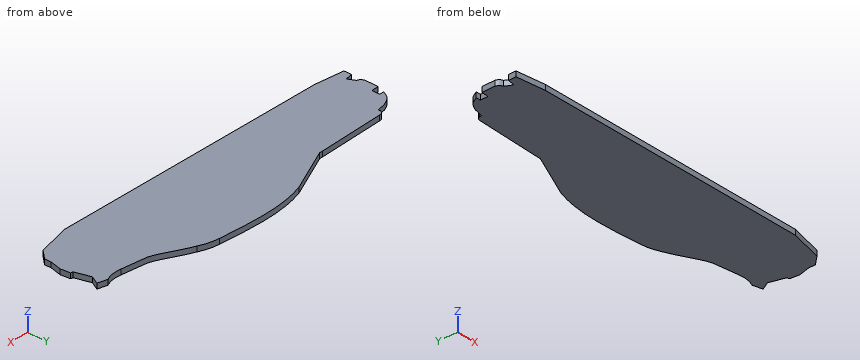
from build123d import *

# Parameters (mm, degrees)
BOSS_EXTRUDE1_DEPTH = 3.18


with BuildPart() as part:
    # Sketch1 → Boss-Extrude1 (new body)
    with BuildSketch(Plane.XY):
        with BuildLine():
            Line((-126.90183157, 63.451351123), (-155.002649134, 50.576))
            Line((-155.002649134, 50.576), (-156.915085055, 50.576))
            Line((-156.915085055, 50.576), (-197.532680285, 48.933631486))
            add(Edge.make_bspline(
                [(-197.532680285, 48.933631486), (-197.856938216, 48.954758252), (-198.175689042, 48.919514289), (-198.799707333, 48.740420096), (-199.089269759, 48.60100182), (-199.619237435, 48.22712778), (-199.847302364, 48.001548224), (-200.130777612, 47.605564254), (-200.213431577, 47.466364131), (-200.354340024, 47.173676097), (-200.419958888, 47.025100819), (-200.487796099, 46.87754919)],
                knots=[0, 0, 0, 0, 0.25, 0.25, 0.5, 0.5, 0.75, 0.75, 0.875, 0.875, 1, 1, 1, 1], degree=3))
            Line((-200.487796099, 46.87754919), (-200.487796099, 45.619190287))
            add(Edge.make_bspline(
                [(-200.487796099, 45.619190287), (-201.175292403, 45.504495406), (-201.855658011, 45.358549214), (-202.871912486, 45.120811128), (-203.209958375, 45.038472689), (-203.885830998, 44.872835338), (-204.223958167, 44.790853124), (-205.235951458, 44.534439775), (-205.906487656, 44.346277621), (-206.874996959, 43.986286634), (-207.191831701, 43.853034452), (-207.811823525, 43.556321951), (-208.418924997, 43.231140141), (-209.00527456, 42.860126187), (-209.584167639, 42.472644028), (-209.869399807, 42.273387637), (-210.694020174, 41.643506759), (-211.201483238, 41.178004532), (-211.73013182, 40.482204306), (-211.831050549, 40.336542937), (-212.018083165, 40.036660904), (-212.101621784, 39.881329534), (-212.681033882, 38.791115208), (-213.177672823, 37.856645785), (-213.674311764, 36.922176363)],
                knots=[0, 0, 0, 0, 0.125, 0.125, 0.1875, 0.1875, 0.25, 0.25, 0.375, 0.375, 0.4375, 0.4375, 0.5, 0.5625, 0.5625, 0.625, 0.625, 0.75, 0.75, 0.78125, 0.78125, 0.8125, 0.8125, 1, 1, 1, 1], degree=3))
            Line((-213.674311764, 36.922176363), (-210.877284017, 36.922176363))
            Line((-210.877284017, 36.922176363), (-210.877284017, 32.540772436))
            add(Edge.make_bspline(
                [(-210.877284017, 32.540772436), (-211.01960291, 32.409346329), (-211.181627568, 32.308403793), (-211.398218963, 32.203976442), (-211.442536276, 32.184489252), (-211.532145699, 32.153014843), (-211.577730345, 32.141242749), (-211.715600825, 32.111602843), (-211.80902927, 32.099543954), (-212.09120418, 32.072973702), (-212.281306192, 32.068469044), (-212.660362358, 32.06338607), (-212.849968469, 32.063384257), (-213.229001172, 32.057537609), (-213.418366995, 32.04971484), (-214.175802907, 32.017532543), (-214.743879841, 31.99339582), (-215.311956775, 31.969259097)],
                knots=[0, 0, 0, 0, 0.125, 0.125, 0.15625, 0.15625, 0.1875, 0.1875, 0.25, 0.25, 0.375, 0.375, 0.5, 0.5, 0.625, 0.625, 1, 1, 1, 1], degree=3))
            Line((-215.311956775, 31.969259097), (-215.311956775, 23.771206966))
            add(Edge.make_bspline(
                [(-215.311956775, 23.771206966), (-215.252651766, 23.614087197), (-215.195691348, 23.455737729), (-215.069051829, 23.145447933), (-214.998440356, 22.994452742), (-214.840114463, 22.702195632), (-214.75241985, 22.56092244), (-214.557151858, 22.289689045), (-214.448883791, 22.159284686), (-214.102194357, 21.800368316), (-213.838466215, 21.600407707), (-213.3989114, 21.353484525), (-213.247390183, 21.281360686), (-212.937649457, 21.155492936), (-212.778720347, 21.102500321), (-212.618220712, 21.053354457)],
                knots=[0, 0, 0, 0, 0.125, 0.125, 0.25, 0.25, 0.375, 0.375, 0.5, 0.5, 0.75, 0.75, 0.875, 0.875, 1, 1, 1, 1], degree=3))
            Line((-212.618220712, 21.053354457), (-210.413324841, 16.852708496))
            Line((-210.413324841, 16.852708496), (-214.842666667, 15.890688618))
            Line((-214.842666667, 15.890688618), (-214.842666667, 11.337489634))
            Line((-214.842666667, 11.337489634), (-197.102804327, 9.286029209))
            Line((-197.102804327, 9.286029209), (-28.009214442, 8.739519054))
            Line((-28.009214442, 8.739519054), (-8.008995649, 13.571514777))
            Line((-8.008995649, 13.571514777), (-3.000125196, 19.110373285))
            Line((-3.000125196, 19.110373285), (-3.000125196, 23.150277734))
            Line((-3.000125196, 23.150277734), (-1.385458215, 30.1458802))
            Line((-1.385458215, 30.1458802), (-1.963054434, 35.965465751))
            Line((-1.963054434, 35.965465751), (-3.410277854, 36.299501866))
            Line((-3.410277854, 36.299501866), (-6.15958565, 45.672965506))
            Line((-6.15958565, 45.672965506), (-3.451467886, 50.891534117))
            Line((-3.451467886, 50.891534117), (-9.2540276, 52.359494102))
            add(Edge.make_bspline(
                [(-9.2540276, 52.359494102), (-9.668938039, 52.177193353), (-10.082311797, 51.990757567), (-10.923946882, 51.657946755), (-11.350787182, 51.507747905), (-12.21693651, 51.240902135), (-12.656745199, 51.124231149), (-13.541049299, 50.927055953), (-13.986464066, 50.846222), (-14.883749808, 50.719684722), (-15.336640435, 50.673980514), (-16.239784909, 50.617569956), (-16.690860317, 50.606663408), (-18.042684657, 50.622754962), (-18.942033937, 50.698486568), (-19.839725309, 50.831943658)],
                knots=[0, 0, 0, 0, 0.125, 0.125, 0.25, 0.25, 0.375, 0.375, 0.5, 0.5, 0.625, 0.625, 0.75, 0.75, 1, 1, 1, 1], degree=3))
            add(Edge.make_bspline(
                [(-19.839725309, 50.831943658), (-23.196389637, 51.361628621), (-26.571655772, 51.738977688), (-30.372384718, 52.134386137), (-30.794736233, 52.177924879), (-31.639473894, 52.264718753), (-32.062038009, 52.307465354), (-33.326315143, 52.447060744), (-34.164847593, 52.554482825), (-35.806204141, 52.888039932), (-36.604486091, 53.1292754), (-38.181447383, 53.676915497), (-38.958811115, 53.987693889), (-41.268211651, 54.995464511), (-42.778587948, 55.7679407), (-45.783734721, 57.329402218), (-47.281168214, 58.120620227), (-51.793167154, 60.454082238), (-54.828124104, 61.954720164), (-57.978327556, 63.220213351)],
                knots=[0, 0, 0, 0, 0.25, 0.25, 0.28125, 0.28125, 0.3125, 0.3125, 0.375, 0.375, 0.4375, 0.4375, 0.5, 0.5, 0.625, 0.625, 0.75, 0.75, 1, 1, 1, 1], degree=3))
            add(Edge.make_bspline(
                [(-57.978327556, 63.220213351), (-59.798164817, 64.087622794), (-61.68095051, 64.789239178), (-65.573057504, 65.841379817), (-67.564024776, 66.185499955), (-69.57343092, 66.350830453)],
                knots=[0, 0, 0, 0, 0.5, 0.5, 1, 1, 1, 1], degree=3))
            add(Edge.make_bspline(
                [(-69.57343092, 66.350830453), (-70.776224616, 66.4631), (-71.980092265, 66.560752996), (-74.387874583, 66.755419067), (-75.591630106, 66.854598111), (-79.20418242, 67.134636215), (-81.61486975, 67.289764959), (-86.440099172, 67.547559017), (-88.853422865, 67.655029171), (-93.681704146, 67.795356063), (-96.096777782, 67.827180782), (-100.929760736, 67.774306212), (-103.340330508, 67.689526026), (-108.134351858, 67.365368434), (-110.519298799, 67.12601353), (-115.259021268, 66.454036055), (-117.613803047, 66.021453535), (-121.118607544, 65.197268693), (-122.282311533, 64.893303875), (-124.599756422, 64.221554126), (-125.753229336, 63.852052568), (-126.90183157, 63.451351123)],
                knots=[0, 0, 0, 0, 0.0625, 0.0625, 0.125, 0.125, 0.25, 0.25, 0.375, 0.375, 0.5, 0.5, 0.625, 0.625, 0.75, 0.75, 0.875, 0.875, 0.9375, 0.9375, 1, 1, 1, 1], degree=3))
        make_face()
    extrude(amount=BOSS_EXTRUDE1_DEPTH)


solid = part.part
Build history of the part. All positions in model axes, mm. Give positions to 0.01 mm unless a question says otherwise; leave off trailing zeros. Write each loop counter-clockwise with the first axis right and the second up, starting at its lowest first coordinate (ties: lowest second). Pieces come first, ordered by that corner, then holes. Notation, with made-up numbers: (61.5, 41) - (92.5, 41) arc R29 ccw to (92.5, 66) - close; hole circle Ø8 at (80.25, -36.5). An arc over 180 degrees is marked (long way). Use one line per item in the form item = value. Start each with the question number.
1. Band-saw the part on B-B on x = -147. Write the cut outline in (y, z).
2. Drop flat-ended pins along their axis: pin 1 Ø1 at (x, z) = (-156.5, 1) entering from +Y; pin 2 Ø1.4 at (x, z) = (-213, 2) entering from -Y; pin 3 Ø1 at (y, z) = (46.5, 1.5) entering from -X; pin 4 Ø5 at (x, y) = (-47, 57.5) entering from -Z. Give the stop position or say it passes through.
3. Band-saw the part on A-A on x = -194. Write the cut outline in (y, z), plus the area to 3 significant figures.
4. Probe line 1 (Y direction, x = -34, z = 0.75); line 2 (Y direction, x = -87.5, z = 1.1); line 3 (X direction, y = 39.5, z = 1.65). List the from-to ranges inside material, lowest first. Write a range as [from, to].
Conclusion:
q1.outline = (9.12, 0) - (54.24, 0) - (54.24, 3.18) - (9.12, 3.18) - close
q2.pin_1 = 50.58
q2.pin_2 = 11.04
q2.pin_3 = -200.49
q2.pin_4 = 0
q3.outline = (9.28, 0) - (49.08, 0) - (49.08, 3.18) - (9.28, 3.18) - close
q3.area = 127 mm²
q4.line_1 = [8.76, 52.55]
q4.line_2 = [8.93, 67.59]
q4.line_3 = [-212.3, -4.35]
